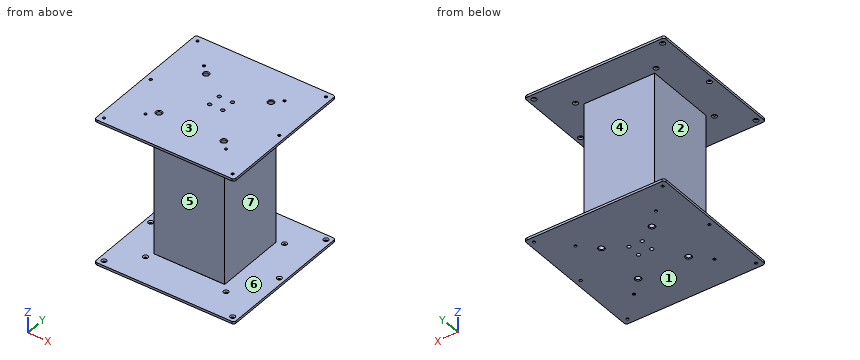
```python
from build123d import *

# Parameters (mm, degrees)
SKETCH1_W           = 295.148
SKETCH1_H           = 295.148
BOSS_EXTRUDE1_DEPTH = 5.08
SKETCH2_W           = 139.192
SKETCH2_H           = 139.192
BOSS_EXTRUDE2_DEPTH = 5.08
SKETCH3_W           = 149.86
SKETCH3_H           = 149.86
BOSS_EXTRUDE3_DEPTH = 294.64
SKETCH4_W           = 295.148
SKETCH4_H           = 295.148
BOSS_EXTRUDE4_DEPTH = 5.08
SKETCH5_R           = 2.794
CUT_EXTRUDE1_DEPTH  = 310.88
CHAMFER1_SIZE       = 2.38
CHAMFER2_SIZE       = 2.38
FILLET1_R           = 5.08
FILLET2_R           = 5.08
SKETCH6_R           = 5.08
CUT_EXTRUDE3_DEPTH  = 35.56
CHAMFER3_SIZE       = 1.524
SKETCH7_R           = 5.08
CUT_EXTRUDE4_DEPTH  = 35.56
CHAMFER5_SIZE       = 1.524
SKETCH8_R           = 3.81
CUT_EXTRUDE5_DEPTH  = 35.56
SKETCH9_R           = 3.81
CUT_EXTRUDE6_DEPTH  = 35.56


with BuildPart() as part:
    # Sketch1 → Boss-Extrude1 (new body)
    with BuildSketch(Plane.XY):
        Rectangle(SKETCH1_W, SKETCH1_H)
    extrude(amount=BOSS_EXTRUDE1_DEPTH)

    # Sketch2 → Boss-Extrude2 (add)
    with BuildSketch(Plane.XY.offset(5.08)):
        Rectangle(SKETCH2_W, SKETCH2_H)
    extrude(amount=BOSS_EXTRUDE2_DEPTH)

    # Sketch3 → Boss-Extrude3 (add)
    with BuildSketch(Plane.XY.offset(10.16)):
        Rectangle(SKETCH3_W, SKETCH3_H)
    extrude(amount=BOSS_EXTRUDE3_DEPTH)

    # Sketch4 → Boss-Extrude4 (add)
    with BuildSketch(Plane.XY.offset(304.8)):
        Rectangle(SKETCH4_W, SKETCH4_H)
    extrude(amount=BOSS_EXTRUDE4_DEPTH)

    # Sketch5 → Cut-Extrude1 (cut, through all)
    with BuildSketch(Plane(origin=(0, 0, 0), x_dir=(-1, 0, 0), z_dir=(0, 0, -1))):
        with Locations((-135.89, 135.89)):
            Circle(SKETCH5_R)
        with Locations((135.89, 135.89)):
            Circle(SKETCH5_R)
        with Locations((135.89, -135.89)):
            Circle(SKETCH5_R)
        with Locations((-135.89, -135.89)):
            Circle(SKETCH5_R)
        with Locations((-135.89, 0)):
            Circle(SKETCH5_R)
        with Locations((135.89, 0)):
            Circle(SKETCH5_R)
        with Locations((-85.09, 85.09)):
            Circle(SKETCH5_R)
        with Locations((85.09, 85.09)):
            Circle(SKETCH5_R)
        with Locations((85.09, -85.09)):
            Circle(SKETCH5_R)
        with Locations((-85.09, -85.09)):
            Circle(SKETCH5_R)
    extrude(amount=-CUT_EXTRUDE1_DEPTH, mode=Mode.SUBTRACT)

    # Chamfer1
    chamfer1_edges = [part.edges().sort_by_distance(p)[0] for p in [
        (138.684, 135.89, 304.8),
    ]]
    chamfer(chamfer1_edges, length=CHAMFER1_SIZE)

    # Chamfer2
    chamfer2_edges = [part.edges().sort_by_distance(p)[0] for p in [
        (138.684, 135.89, 5.08),
        (-133.096, 0, 5.08),
        (-133.096, 0, 304.8),
        (87.884, 85.09, 5.08),
        (87.884, 85.09, 304.8),
        (-82.296, 85.09, 5.08),
        (-82.296, 85.09, 304.8),
        (-82.296, -85.09, 5.08),
        (-82.296, -85.09, 304.8),
        (138.684, 0, 5.08),
        (138.684, 0, 304.8),
        (138.684, -135.89, 5.08),
        (138.684, -135.89, 304.8),
        (-133.096, -135.89, 5.08),
        (-133.096, -135.89, 304.8),
        (-133.096, 135.89, 5.08),
        (-133.096, 135.89, 304.8),
        (87.884, -85.09, 5.08),
        (87.884, -85.09, 304.8),
    ]]
    chamfer(chamfer2_edges, length=CHAMFER2_SIZE)

    # Fillet1
    fillet1_edges = [part.edges().sort_by_distance(p)[0] for p in [
        (147.574, 147.574, 2.54),
    ]]
    fillet(fillet1_edges, radius=FILLET1_R)

    # Fillet2
    fillet2_edges = [part.edges().sort_by_distance(p)[0] for p in [
        (-147.574, 147.574, 307.34),
        (-147.574, -147.574, 307.34),
        (147.574, -147.574, 307.34),
        (147.574, 147.574, 307.34),
        (147.574, -147.574, 2.54),
        (-147.574, -147.574, 2.54),
        (-147.574, 147.574, 2.54),
    ]]
    fillet(fillet2_edges, radius=FILLET2_R)

    # Sketch6 → Cut-Extrude3 (cut)
    with BuildSketch(Plane.XY.offset(309.88)):
        with Locations((-68.58, -68.58)):
            Circle(SKETCH6_R)
        with Locations((-68.58, 68.58)):
            Circle(SKETCH6_R)
        with Locations((68.58, 68.58)):
            Circle(SKETCH6_R)
        with Locations((68.58, -68.58)):
            Circle(SKETCH6_R)
    extrude(amount=-CUT_EXTRUDE3_DEPTH, mode=Mode.SUBTRACT)

    # Chamfer3
    chamfer3_edges = [part.edges().sort_by_distance(p)[0] for p in [
        (63.5, -68.58, 309.88),
        (63.5, 68.58, 309.88),
        (-73.66, 68.58, 309.88),
        (-73.66, -68.58, 309.88),
    ]]
    chamfer(chamfer3_edges, length=CHAMFER3_SIZE)

    # Sketch7 → Cut-Extrude4 (cut)
    with BuildSketch(Plane(origin=(0, 0, 0), x_dir=(-1, 0, 0), z_dir=(0, 0, -1))):
        with Locations((-53.34, 53.34)):
            Circle(SKETCH7_R)
        with Locations((-53.34, -53.34)):
            Circle(SKETCH7_R)
        with Locations((53.34, -53.34)):
            Circle(SKETCH7_R)
        with Locations((53.34, 53.34)):
            Circle(SKETCH7_R)
    extrude(amount=-CUT_EXTRUDE4_DEPTH, mode=Mode.SUBTRACT)

    # Chamfer5
    chamfer5_edges = [part.edges().sort_by_distance(p)[0] for p in [
        (-48.26, 53.34, 0),
        (-48.26, -53.34, 0),
        (58.42, -53.34, 0),
        (58.42, 53.34, 0),
    ]]
    chamfer(chamfer5_edges, length=CHAMFER5_SIZE)

    # Sketch8 → Cut-Extrude5 (cut)
    with BuildSketch(Plane.XY.offset(309.88)):
        with Locations((15.494, 29.464)):
            Circle(SKETCH8_R)
        with Locations((15.494, 1.524)):
            Circle(SKETCH8_R)
        with Locations((-12.446, 1.524)):
            Circle(SKETCH8_R)
        with Locations((-12.446, 29.464)):
            Circle(SKETCH8_R)
    extrude(amount=-CUT_EXTRUDE5_DEPTH, mode=Mode.SUBTRACT)

    # Sketch9 → Cut-Extrude6 (cut)
    with BuildSketch(Plane(origin=(0, 0, 0), x_dir=(-1, 0, 0), z_dir=(0, 0, -1))):
        with Locations((15.494, 29.464)):
            Circle(SKETCH9_R)
        with Locations((15.494, 1.524)):
            Circle(SKETCH9_R)
        with Locations((-12.446, 29.464)):
            Circle(SKETCH9_R)
        with Locations((-12.446, 1.524)):
            Circle(SKETCH9_R)
    extrude(amount=-CUT_EXTRUDE6_DEPTH, mode=Mode.SUBTRACT)


solid = part.part
```
Could you check a few things on this model? Use its own coordinates, in mm. Face numbers are marked on the shaded views. A direction names the side the tool comes from. Round coordinates to 2 decimals unless told otherwise and drop trailing zeros. Loops run counter-clockwise (first coordinate to the right, second up) from the corner with the lowest first, then second, coordinate; pieces in that order, holes last. Notation, with made-up numbers: (3.5, 48.5) - (35.5, 48.5) arc R18 ccw to (35.5, 82.5) - close; hole circle Ø2 at (16.25, -6). An arc over 180 degrees is marked (long way). Use CSV: the item, a comma, the result in double quotes.
Item 1: For the marked faces 4, 5, 6 and 7, which set-ups out of +Z, -Z, +X, -X, +Y, -Y let a thin tool reach every point of the face, with its end or its side?
Here are the results:
face 4,"+X, -X, +Y"
face 5,"+X, -X, -Y"
face 6,"none"
face 7,"+X, +Y, -Y"
Item 2: If we section it at C-C on z = 27: Count the separate pieces of the cut face and the enclosed holes in it, then the cut area to 3 significant figures.
Here are the results:
separate pieces,"1"
enclosed holes,"8"
area,"22,000 mm²"
Item 3: If we section it at B-B on y = -42.5: List the corners of the cut face in (x, z) for me, then the cut area to 3 significant figures.
Here are the results:
outline,"(-147.57, 0) - (147.57, 0) - (147.57, 5.08) - (69.6, 5.08) - (69.6, 10.16) - (74.93, 10.16) - (74.93, 304.8) - (147.57, 304.8) - (147.57, 309.88) - (-147.57, 309.88) - (-147.57, 304.8) - (-74.93, 304.8) - (-74.93, 10.16) - (-69.6, 10.16) - (-69.6, 5.08) - (-147.57, 5.08) - close"
area,"47,900 mm²"
Item 4: If we mould it in two halves opening along Z, with no side actions, what happens to the marked faces 1, 2 and 3? For each: pulls with the +Z half, pulls with the -Z half, needs draft (parallel to the pull), parting line crosses it, or undercut.
Here are the results:
face 1,"pulls with the -Z half"
face 2,"undercut"
face 3,"pulls with the +Z half"
Item 5: If we section it at A-A on x = 101: List the corners of the cut face in (y, z) for me, then the cut area to 3 significant figures.
Here are the results:
outline,"(-147.57, 0) - (147.57, 0) - (147.57, 5.08) - (-147.57, 5.08) - close; (-147.57, 304.8) - (147.57, 304.8) - (147.57, 309.88) - (-147.57, 309.88) - close"
area,"3,000 mm²"
Item 6: Will these pins go through, and if not, where does the flat tip stop? pin 1 (4 mm diameter, centred on x = -26, z = 8, fed in from -Y); pin 2 (5 mm diameter, centred on x = 56, y = 51.5, fed in from -Z); pin 3 (12 mm diameter, centred on x = 29.5, z = 108, fed in from +Y).
Here are the results:
pin 1,"stops at y = -69.6"
pin 2,"stops at z = 0.87"
pin 3,"stops at y = 74.93"
Item 7: I need wall thicknesses on L1, parallel to X at y = -135.89, z = 308.1; L2, parallel to Y at x = -85.09, z = 1.4; L3, parallel to Z at x = 30, y = 75. Which ranges of each line are inside material? Lowest first, please. Write a range as [from, to].
Here are the results:
L1,"x = [-147.57, -138.68], [-133.1, 133.1], [138.68, 147.57]"
L2,"y = [-147.57, -87.88], [-82.3, 82.3], [87.88, 147.57]"
L3,"z = [0, 5.08], [304.8, 309.88]"
